from build123d import *

# Parameters (mm, degrees)
F0_R     = 3.175
F1_DEPTH = 3.175
F3_R     = 1.016


with BuildPart() as f1:
    # F0 (on Front) → F1 (new body)
    with BuildSketch(Plane.XZ):
        with BuildLine():
            ThreePointArc((151.351172, 102.087654), (161.19312, -85.707902), (0, -182.5625))
            Line((0, -182.5625), (0, -273.3929))
            Line((0, -273.3929), (230.726172, -273.3929))
            Line((230.726172, -273.3929), (230.726172, -182.5625))
            Line((230.726172, -182.5625), (230.726172, 102.087654))
            Line((230.726172, 102.087654), (151.351172, 102.087654))
        make_face()
        with BuildLine():
            ThreePointArc((131.587777, -138.5951), (131.773765, -138.146087), (132.222777, -137.9601))
            Line((132.222777, -137.9601), (177.942777, -137.9601))
            ThreePointArc((177.942777, -137.9601), (178.39179, -138.146087), (178.577777, -138.5951))
            Line((178.577777, -138.5951), (178.577777, -182.5625))
            Line((178.577777, -182.5625), (131.587777, -182.5625))
            Line((131.587777, -182.5625), (131.587777, -138.5951))
        make_face(mode=Mode.SUBTRACT)
        with Locations((211.676172, -106.3625)):
            Circle(F0_R, mode=Mode.SUBTRACT)
        with Locations((211.676172, 25.887654)):
            Circle(F0_R, mode=Mode.SUBTRACT)
    extrude(amount=F1_DEPTH)

    # F3
    f3_edges = [f1.edges().sort_by_distance(p)[0] for p in [
        (151.351172, -1.5875, 102.087654),
        (0, -1.5875, -182.5625),
    ]]
    fillet(f3_edges, radius=F3_R)


solid = f1.part
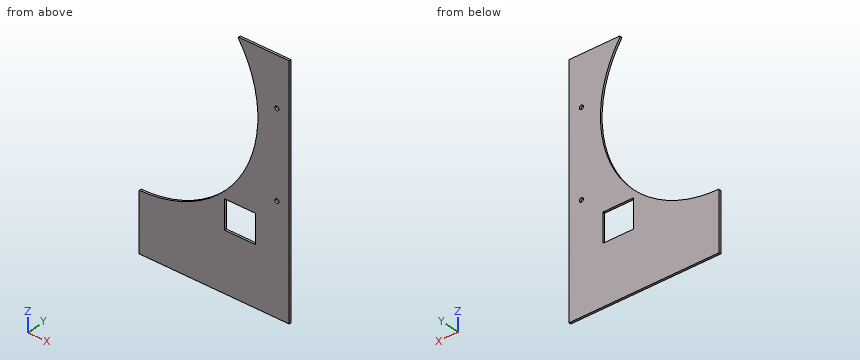
Build history of the part. All positions in model axes, mm. Round coordinates to 2 decimals unless told otherwise and drop trailing zeros. Write each loop counter-clockwise with the first axis right and the second up, starting at its lowest first coordinate (ties: lowest second). Pieces come first, ordered by that corner, then holes. Notation, with made-up numbers: M 17,43.5 L 55,43.5 A19 ccw 55,51.5 Z; hole C -39.75,41 d1. An arc over 180 degrees is marked long. Answer as a JSON object with one key per item and string values. Group by question number.
(1) Cut at C-C (z = -162.5). Give the cut face in (x, y) (3 decimals).
(2) Flat gauge pins, fed straight in: pin 1 (1.5 mm diameter, centred on y = -3, z = 57.5, fed in from -X); pin 2 (7.5 mm diameter, centred on x = 211.68, z = -106.36, fed in from +Y); pin 3 (1.6 mm diameter, centred on y = -2.5, z = -164.5, fed in from -X). Where does each tip first touch, or does it go through?
(3) Cut at A-A (x = 140). Give the cut face in (y, z) (1 decimal).
(4) Drill centre lines: L1, parallel to Z at x = 210, y = -1.25; L2, parallel to Z at x = 142.5, y = -2.1; L3, parallel to X at y = -0.15, z = 3.5. Where is each one in solid material? Low to high.
(5) Cut at D-D (x = 164). Give the cut face in (y, z) (1 decimal), and give its area (3 significant figures).
(6) Cut at B-B (y = -1.1). Give the number of separate pieces and of enclosed holes in the cut face, and give its area (3 significant figures).
Responses:
{
 "1": {"outline": "M 83.203,-3.175 L 131.588,-3.175 L 131.588,0 L 83.203,0 Z; M 178.578,-3.175 L 230.726,-3.175 L 230.726,0 L 178.578,0 Z"},
 "2": {"pin 1": "stops at x = 173.02", "pin 2": "stops at y = 0", "pin 3": "stops at x = 77.49"},
 "3": {"outline": "M -3.2,-273.4 L 0,-273.4 L 0,-182.6 L -3.2,-182.6 Z; M -3.2,-138 L 0,-138 L 0,-117.2 L -3.2,-117.2 Z"},
 "4": {"L1": "z = -273.39 to -109.06, -103.67 to 23.19, 28.58 to 102.09", "L2": "z = -273.39 to -182.56, -137.96 to -114.12", "L3": "x = 182.53 to 230.73"},
 "5": {"outline": "M -3.2,-273.4 L 0,-273.4 L 0,-182.6 L -3.2,-182.6 Z; M -3.2,-138 L 0,-138 L 0,-80.2 L -3.2,-80.2 Z; M -3.2,80.2 L 0,80.2 L 0,102.1 L -3.2,102.1 Z", "area": "541 mm2"},
 "6": {"separate pieces": "1", "enclosed holes": "3", "area": "40,700 mm2"}
}
